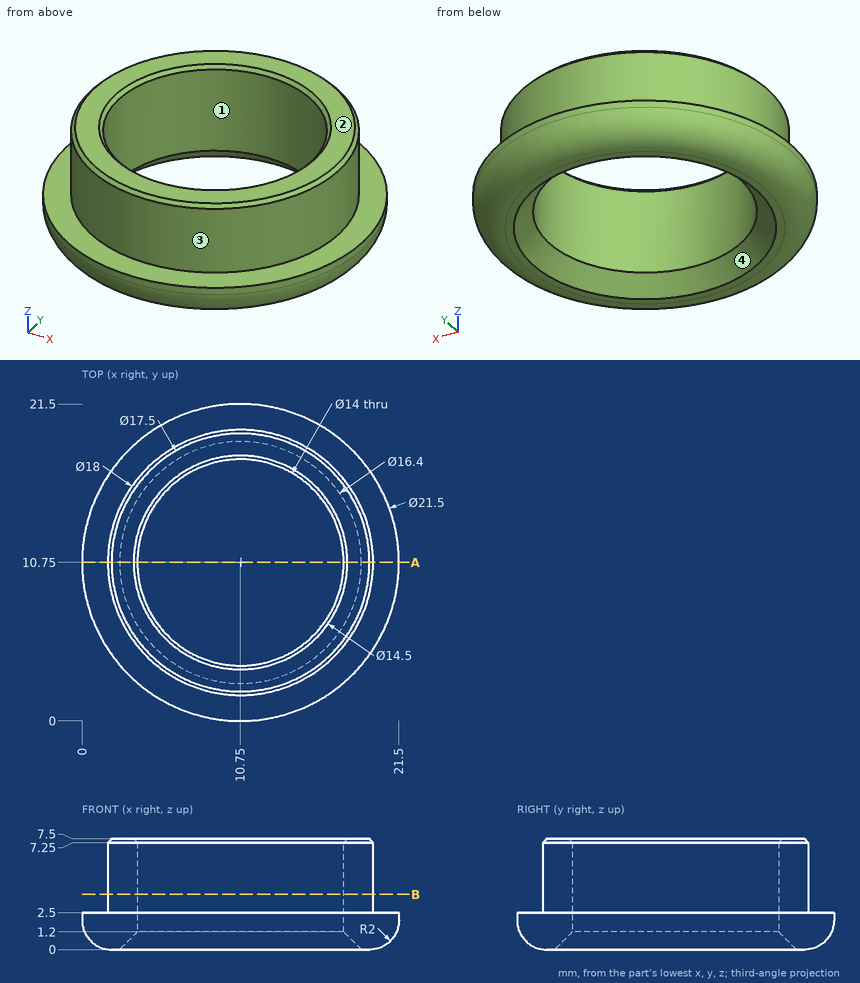
Design review of the part shown in the three views and the two pictorial views. Dimensions are in mm from the part's minimum x, y and z. Round coordinates to 2 decimals unless told otherwise and drop trailing zeros. Order: outer loops, then holes, each group sorted by start corner. A loop starts at its lowest first (then second) coordinate and runs counter-clockwise, first axis right, second up. Notation, with made-up numbers: M 26,-31.5 L 77,-31.5 A9 ccw 77,-21.5 Z; hole C -33,-30 d4. An arc over 180 degrees is marked long. Put each result on its own line as item: value.
Q1. Draft analysis for pull direction X (two halves, no side actions). For the marked faces 1, 2, 3 and 4, state which applies: released by +X, released by -X, zero draft, split by the parting line, or undercut.
Reported:
face 1: undercut
face 2: zero draft
face 3: split by the parting line
face 4: undercut
Q2. To check wall thickness, follow line 1 (Y direction, x = 10.75, z = 4); line 2 (Y direction, x = 4.5, z = 0.75); line 3 (X direction, y = 12.25, z = 6.5). State the ranges of each line that lie inside material, in increasing order.
Reported:
line 1: 1.75 to 3.75, 17.75 to 19.75
line 2: 2.55 to 6.7, 14.8 to 18.95
line 3: 1.88 to 3.91, 17.59 to 19.62
Q3. Insertion check: pin 1 Ø2 at (y, z) = (6, 2) entering from +X; pin 2 Ø8 at (x, y) = (10, 16) entering from +Z; pin 3 Ø1 at (x, z) = (4.5, 3.5) entering from +Y; pin 4 Ø1 at (x, z) = (7.5, 1.5) entering from -Y. Each pin has a flat end and moves straight along its axis. Give the tip position at first contact, or say it passes through.
Reported:
pin 1: x = 20.82
pin 2: z = 7.5
pin 3: y = 17.67
pin 4: y = 0.39
Q4. Consider section B-B (z = 3.75). State the section outline as (x, y) points.
Reported:
outline: C 10.75,10.75 d18; hole C 10.75,10.75 d14
Q5. Consider section A-A (y = 10.75). State the section outline as (x, z) points, and give its area (3 significant figures).
Reported:
outline: M 0,2 A2 ccw 2,0 L 2.55,0 L 3.75,1.2 L 3.75,7.25 L 3.5,7.5 L 2,7.5 L 1.75,7.25 L 1.75,2.5 L 0,2.5 Z; M 17.75,1.2 L 18.95,0 L 19.5,0 A2 ccw 21.5,2 L 21.5,2.5 L 19.75,2.5 L 19.75,7.25 L 19.5,7.5 L 18,7.5 L 17.75,7.25 Z
area: 35.5 mm²
